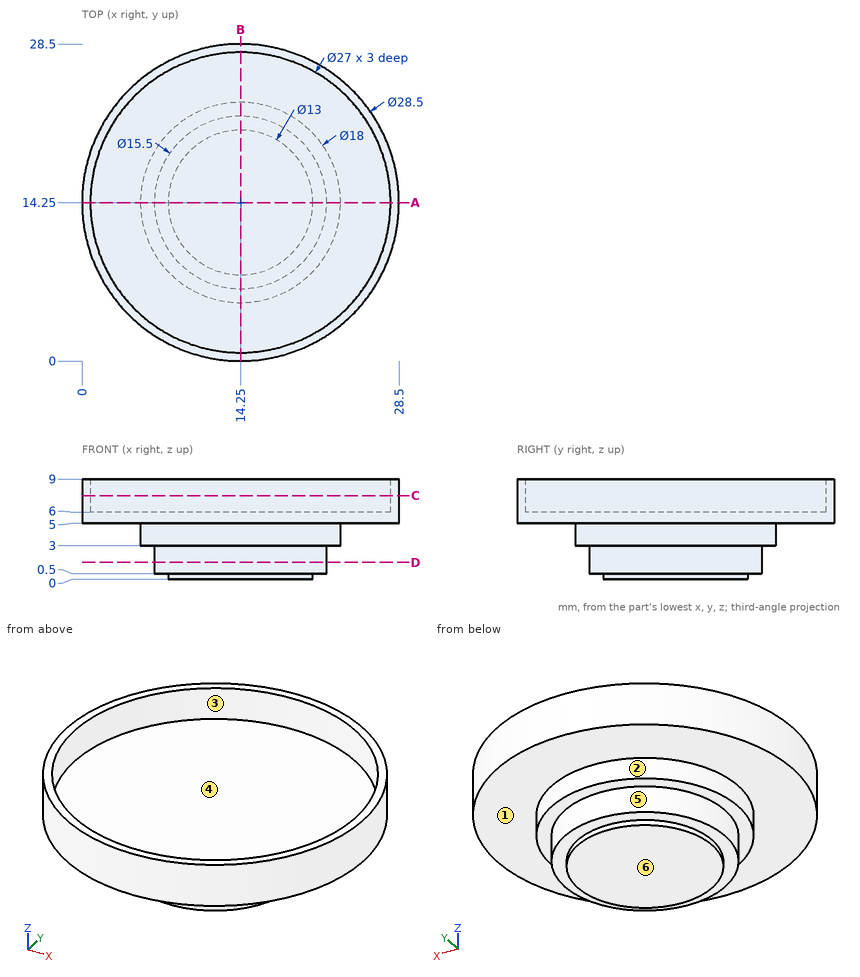
Here's the drawing with two shaded views (mm, measured from the low corner). I have some questions. A direction names the side the tool comes from. Give positions to 0.01 mm unless a question says otherwise; leave off trailing zeros. Loops run counter-clockwise (first coordinate to the right, second up) from the corner with the lowest first, then second, coordinate; pieces in that order, holes last. Notation, with made-up numbers: M -14,46.25 L 39,46.25 A36 ccw 39,84.25 Z; hole C 73.25,10.5 d3. An arc over 180 degrees is marked long. One line per item, written item: value. Start each with the question number.
1) If we section it at C-C, the plane z = 7.5: Write out the boundary of the cut face in (x, y), and give its area (3 significant figures).
2) Thinking about a two-plate mould opening in X: for the marked faces 1, 2 and 3, which applies, +X half, -X half, draft (parallel to the pull), parting line (faces both ways), or undercut?
3) I'm going to push flat-ended pins straight in: pin 1 (2 mm diameter, centred on x = 12, z = 1.5, fed in from +Y); pin 2 (1.5 mm diameter, centred on x = 14.5, y = 18, fed in from +Z); pin 3 (2 mm diameter, centred on y = 21.5, z = 2.5, fed in from -X). Where does each tip first touch, or does it pass through?
4) If we section it at D-D, the plane z = 1.5: Write out the boundary of the cut face in (x, y), and give its area (3 significant figures).
5) If I drill on line 1 (Y direction, x = 14.25, z = 6.9); line 2 (Z direction, x = 23.25, y = 24.25); line 3 (Y direction, x = 12.5, z = 8), over which ranges is the centre line in solid material (lowest first)? Write a range as [from, to].
6) On a 3-axis mill with a long thin cutter (end or side, diameter ignored), from which of +Z, -Z, +X, -X, +Y, -Y can I reach the whole of each face in a straight line? I mean the marked faces 4, 5 and 6. Say none if no direction works.
7) If we section it at A-A, the plane y = 14.25: Write out the boundary of the cut face in (x, z).
Completed:
1. outline: C 14.25,14.25 d28.5; hole C 14.25,14.25 d27
1. area: 65.4 mm^2
2. face 1: draft
2. face 2: parting line
2. face 3: undercut
3. pin 1: stops at y = 21.9
3. pin 2: stops at z = 6
3. pin 3: stops at x = 7.91
4. outline: C 14.25,14.25 d15.5
4. area: 189 mm^2
5. line 1: y = [0, 0.75], [27.75, 28.5]
5. line 2: z = [5, 6]
5. line 3: y = [0.11, 0.86], [27.64, 28.39]
6. face 4: +Z
6. face 5: -Z
6. face 6: -Z, +X, -X, +Y, -Y
7. outline: M 0,5 L 5.25,5 L 5.25,3 L 6.5,3 L 6.5,0.5 L 7.75,0.5 L 7.75,0 L 20.75,0 L 20.75,0.5 L 22,0.5 L 22,3 L 23.25,3 L 23.25,5 L 28.5,5 L 28.5,9 L 27.75,9 L 27.75,6 L 0.75,6 L 0.75,9 L 0,9 Z
